Verification items for the finished model (mm, model axes). Face numbers are marked on the shaded views. Coordinates: 2 decimals unless noted, no trailing zeros. Write each loop counter-clockwise with the first axis right and the second up, starting at its lowest first coordinate (ties: lowest second). Pieces come first, ordered by that corner, then holes.
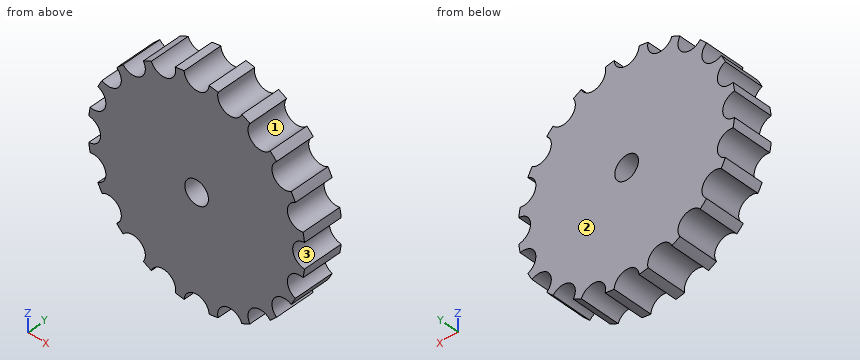
```python
from build123d import *

# Parameters (mm, degrees)
F0_R            = 27.5
F0_R_2          = 3
F1_DEPTH        = 10
F2_R            = 3.17
F3_DEPTH        = 10.001
F3_COPIES_COUNT = 20


# Not quite as in the source:
# - a pattern or mirror of a feature is missing from the dataset's text; its kind, count and spacing are read off the source's solid


with BuildPart() as f1:
    # F0 (on Front) → F1 (new body)
    with BuildSketch(Plane.XZ):
        Circle(F0_R)
        Circle(F0_R_2, mode=Mode.SUBTRACT)
    extrude(amount=F1_DEPTH)

    # F2 (on face) → F3 (cut, through all)
    with BuildSketch(Plane.XZ.offset(10)):
        with Locations((0, 27.5)):
            Circle(F2_R)
    f3 = extrude(amount=-F3_DEPTH, mode=Mode.SUBTRACT)

    # F3_copies: F3 ×20 about axis
    f3_copies_axis = Axis((0, 0, 0), (0, 1, 0))
    for i in range(1, F3_COPIES_COUNT):
        add(f3.rotate(f3_copies_axis, i * 360 / F3_COPIES_COUNT), mode=Mode.SUBTRACT)


solid = f1.part
```
1. Gauge pin test, flat ends, axial feed: P1, Ø2, axis at y = -3, z = -1, coming from the +X side; P2, Ø2, axis at y = -3.5, z = 19, coming from the +X side. Record the tip position at first contact, or that the pin passes through.
2. Sectioned sample at A-A, the plane z = 0. Record the boundary of the cut face in (x, y), and give its area (3 significant figures).
3. Material ranges on L1, parallel to Z at x = 0, y = -7.25; L2, parallel to Z at x = 19.5, y = -4.75; L3, parallel to Z at x = -16, y = -5.5, recorded low to high.
4. Sectioned sample at B-B, the plane x = 0. Record the boundary of the cut face in (y, z), and give its area (3 significant figures).
5. Draft check along X on the marked faces 1, 2 and 3. Enter one of: pulls with the +X half, pulls with the -X half, needs draft (parallel to the pull), parting line crosses it, or undercut.
Outcome:
1. P1: stops at x = 25.04
1. P2: stops at x = 20.24
2. outline: (-24.33, -10) - (-3, -10) - (-3, 0) - (-24.33, 0) - close; (3, -10) - (24.33, -10) - (24.33, 0) - (3, 0) - close
2. area: 427 mm2
3. L1: z = -24.33 to -3, 3 to 24.33
3. L2: z = -19.39 to -17.74, -14.58 to 14.58, 17.74 to 19.39
3. L3: z = -19.08 to 19.08
4. outline: (-10, -24.33) - (0, -24.33) - (0, -3) - (-10, -3) - close; (-10, 3) - (0, 3) - (0, 24.33) - (-10, 24.33) - close
4. area: 427 mm2
5. face 1: undercut
5. face 2: needs draft
5. face 3: pulls with the +X half
